from build123d import *

# Parameters (mm, degrees)
SKETCH_1_W      = 30
SKETCH_1_H      = 14
EXTRUDE_1_DEPTH = 8
SKETCH_2_R      = 0.35
EXTRUDE_2_DEPTH = 2


with BuildPart() as part:
    # 草图1 → 凸台-拉伸1 (new body)
    with BuildSketch(Plane.XY):
        with Locations((15, 7)):
            Rectangle(SKETCH_1_W, SKETCH_1_H)
    extrude(amount=EXTRUDE_1_DEPTH)

    # 草图2 → 凸台-拉伸2 (add)
    with BuildSketch(Plane.XY.offset(8)):
        with Locations(Location((13.73, 12, 0), (0, 0, 180))):
            Circle(SKETCH_2_R)
        with Locations(Location((16.27, 12, 0), (0, 0, 180))):
            Circle(SKETCH_2_R)
        with Locations(Location((18.81, 12, 0), (0, 0, 180))):
            Circle(SKETCH_2_R)
        with Locations(Location((21.35, 12, 0), (0, 0, 180))):
            Circle(SKETCH_2_R)
        with Locations(Location((13.73, 2, 0), (0, 0, 180))):
            Circle(SKETCH_2_R)
        with Locations(Location((16.27, 2, 0), (0, 0, 180))):
            Circle(SKETCH_2_R)
        with Locations(Location((18.81, 2, 0), (0, 0, 180))):
            Circle(SKETCH_2_R)
        with Locations(Location((21.35, 2, 0), (0, 0, 180))):
            Circle(SKETCH_2_R)
        with Locations(Location((11.19, 12, 0), (0, 0, 180))):
            Circle(SKETCH_2_R)
        with Locations(Location((8.65, 12, 0), (0, 0, 180))):
            Circle(SKETCH_2_R)
        with Locations(Location((11.19, 2, 0), (0, 0, 180))):
            Circle(SKETCH_2_R)
        with Locations(Location((8.65, 2, 0), (0, 0, 180))):
            Circle(SKETCH_2_R)
    extrude(amount=EXTRUDE_2_DEPTH)


solid = part.part
Design review of the part built by this model. Coordinates are the model's own, in mm. Round coordinates to 2 decimals unless told otherwise and drop trailing zeros. Order: outer loops, then holes, each group sorted by start corner. A loop starts at its lowest first (then second) coordinate and runs counter-clockwise, first axis right, second up.
1) Clearance check with a flat-ended pin moving along its axis: pin 1 Ø7 at (x, y) = (21.5, 6) entering from +Z. State where the tip first meets the part, or that it passes through.
The answers:
pin 1: stops at z = 8
2) For L1, parallel to Z at x = 3.75, y = 8.5, list the stretches that pass through material, from the lowest coordinate up.
The answers:
L1: z = 0 to 8
3) Consider section C-C (x = 13). State the section outline as (y, z) points.
The answers:
outline: (0, 0) - (14, 0) - (14, 8) - (0, 8) - close
4) Consider section A-A (x = 8.65). State the section outline as (y, z) points.
The answers:
outline: (0, 0) - (14, 0) - (14, 8) - (12.35, 8) - (12.35, 10) - (11.65, 10) - (11.65, 8) - (2.35, 8) - (2.35, 10) - (1.65, 10) - (1.65, 8) - (0, 8) - close
5) Consider section B-B (y = 3.75). State the section outline as (x, z) points, plus the area to 3 significant figures.
The answers:
outline: (0, 0) - (30, 0) - (30, 8) - (0, 8) - close
area: 240 mm2
